Autodesk Inventor part; units mm, degrees
ref_plane "YZ Plane" through (0, 0, 0) normal (1, 0, 0) x (0, 1, 0)
ref_plane "XZ Plane" through (0, 0, 0) normal (0, 1, 0) x (-1, 0, 0)
ref_plane "XY Plane" through (0, 0, 0) normal (0, 0, 1) x (1, 0, 0)
sketch "Sketch1" plane through (0, 0, 0) normal (0, 1, 0) x (-1, 0, 0)
  line L0 (44.45, 203.2) -> (-44.45, 203.2)
  line L1 (-44.45, 203.2) -> (-44.45, -203.2)
  line L2 (-44.45, -203.2) -> (44.45, -203.2)
  line L3 (44.45, -203.2) -> (44.45, 203.2)
  line L4 (44.45, 203.2) -> (-44.45, -203.2) construction
  line L5 (-44.45, 203.2) -> (44.45, -203.2) construction
  line L6 (-44.45, 203.2) -> (-20.955, 203.2)
  line L7 (-20.955, 203.2) -> (-20.955, 88.9) construction
  line L8 (-44.45, 88.9) -> (-44.45, 203.2)
  circle A0 centre (-20.955, 88.9) radius 15.494 construction
  line L9 (44.45, 203.2) -> (44.45, 111.6492)
  line L10 (44.45, 203.2) -> (44.45, 38.1)
  line L11 (44.45, 38.1) -> (22.225, 38.1) construction
  circle A1 centre (22.225, 38.1) radius 12.065 construction
  line L12 (-66.675, 88.9) -> (0, 88.9) construction
  line L13 (0, 88.9) -> (0, 203.2) construction
  line L14 (0, 203.2) -> (-66.675, 203.2)
  line L15 (-66.675, 203.2) -> (-66.675, 88.9) construction
  line L16 (-66.675, 203.2) -> (-66.675, 209.55) construction
  line L17 (-66.675, 209.55) -> (32.5679, 44.312) construction
  circle A2 centre (-20.955, 104.394) radius 1.5
  circle A3 centre (-34.3732, 96.647) radius 1.5
  circle A4 centre (-34.3732, 81.153) radius 1.5
  circle A5 centre (-20.955, 73.406) radius 1.5
  circle A6 centre (-7.5368, 81.153) radius 1.5
  circle A7 centre (-7.5368, 96.647) radius 1.5
  circle A8 centre (-20.955, 88.9) radius 7.112 construction
  circle A9 centre (-28.067, 88.9) radius 5.9944
  line L18 (-20.955, 88.9) -> (-20.955, 152.4) construction
  circle A10 centre (-20.955, 152.4) radius 8.001 construction
  circle A11 centre (-20.955, 152.4) radius 4.0005
  circle A12 centre (-20.955, 160.401) radius 1.85
  line L19 (42.545, 152.4) -> (-20.955, 152.4) construction
  circle A13 centre (-28.956, 152.4) radius 1.85
  line L20 (-20.955, 215.9) -> (-20.955, 152.4) construction
  circle A14 centre (-20.955, 144.399) radius 1.85
  line L21 (-84.455, 152.4) -> (-20.955, 152.4) construction
  circle A15 centre (-12.954, 152.4) radius 1.85
  line L22 (44.45, 0) -> (-44.45, 0) construction
  circle A16 centre (22.225, 38.1) radius 2.9766
  circle A17 centre (22.225, -38.1) radius 2.9766
  circle A18 centre (-33.8743, 119.8397) radius 12.065 construction
  circle A19 centre (-33.8743, 119.8397) radius 2.9766
  circle A20 centre (-20.955, 152.4) radius 50.8 construction
  line L23 (32.5679, 44.312) -> (22.7595, 60.6429) construction
  line L24 (22.7595, 60.6429) -> (17.8553, 68.8083) construction
  line L25 (15.6729, 78.6085) -> (25.4813, 62.2776)
  line L26 (25.4813, 62.2776) -> (20.0377, 59.0081)
  line L27 (20.0377, 59.0081) -> (10.2292, 75.339)
  line L28 (10.2292, 75.339) -> (15.6729, 78.6085)
  line L29 (15.6729, 78.6085) -> (20.0377, 59.0081) construction
  line L30 (25.4813, 62.2776) -> (10.2292, 75.339) construction
  line L31 (-3.944, 111.2702) -> (5.8645, 94.9394)
  line L32 (-9.3876, 108.0008) -> (-3.944, 111.2702)
  line L33 (5.8645, 94.9394) -> (0.4208, 91.6699)
  line L34 (0.4208, 91.6699) -> (-9.3876, 108.0008)
  line L35 (-23.5608, 143.932) -> (-13.7524, 127.6011)
  line L36 (-29.0044, 140.6625) -> (-23.5608, 143.932)
  line L37 (-13.7524, 127.6011) -> (-19.196, 124.3316)
  line L38 (-19.196, 124.3316) -> (-29.0044, 140.6625)
  circle A21 centre (-20.955, -104.394) radius 1.5
  circle A22 centre (-34.3732, -81.153) radius 1.5
  circle A23 centre (-7.5368, -81.153) radius 1.5
  circle A24 centre (-28.067, -88.9) radius 5.9944
  circle A25 centre (-20.955, -152.4) radius 4.0005
  circle A26 centre (-28.956, -152.4) radius 1.85
  circle A27 centre (-12.954, -152.4) radius 1.85
  circle A28 centre (22.225, -38.1) radius 2.9766
  circle A29 centre (-33.8743, -119.8397) radius 2.9766
  circle A30 centre (-29.2932, -53.9743) radius 3.175
  circle A31 centre (-28.067, 88.9) radius 31.75 construction
  line L39 (-28.067, 88.9) -> (-44.45, 88.9) construction
  line L40 (-44.45, 88.9) -> (-44.45, 12.7)
  line L41 (44.45, 203.2) -> (34.925, 203.2)
  line L42 (34.925, 203.2) -> (34.925, 193.675) construction
  line L43 (34.925, 193.675) -> (44.45, 193.675) construction
  line L44 (44.45, 193.675) -> (44.45, 203.2)
  circle A32 centre (34.925, 193.675) radius 3.175
  line L45 (-44.45, 0) -> (-31.75, 0)
  circle A33 centre (-31.75, 0) radius 3.175
  circle A34 centre (34.925, -193.675) radius 3.175
  line L46 (-44.45, 0) -> (-19.455, 0) construction
  line L47 (-16.28, -76.0639) -> (-22.63, -76.0639) construction
  line L48 (-22.63, -76.0639) -> (-22.63, 51.9267) construction
  line L49 (-22.63, 51.9267) -> (-16.28, 51.9267) construction
  line L50 (-16.28, 51.9267) -> (-16.28, -76.0639) construction
  line L51 (-16.28, -63.9953) -> (-22.63, 63.9953) construction
  line L52 (-22.63, -63.9953) -> (-16.28, 63.9953) construction
  line L53 (-16.28, 51.9267) -> (-22.63, -76.0639) construction
  line L54 (-22.63, 51.9267) -> (-16.28, -76.0639) construction
  line L55 (-16.28, -2.5436) -> (-22.63, -2.5436)
  line L56 (-22.63, -2.5436) -> (-22.63, -21.5936)
  line L57 (-22.63, -21.5936) -> (-16.28, -21.5936)
  line L58 (-16.28, -21.5936) -> (-16.28, -2.5436)
  line L59 (-16.28, -2.5436) -> (-22.63, -21.5936) construction
  line L60 (-22.63, -2.5436) -> (-16.28, -21.5936) construction
  line L61 (-16.28, -40.6436) -> (-22.63, -40.6436)
  line L62 (-16.28, -59.6936) -> (-16.28, -40.6436)
  line L63 (-22.63, -40.6436) -> (-22.63, -59.6936)
  line L64 (-22.63, -59.6936) -> (-16.28, -59.6936)
  line L65 (-16.28, 35.5564) -> (-22.63, 35.5564)
  line L66 (-16.28, 16.5064) -> (-16.28, 35.5564)
  line L67 (-22.63, 35.5564) -> (-22.63, 16.5064)
  line L68 (-22.63, 16.5064) -> (-16.28, 16.5064)
  line L69 (-16.28, -2.5436) -> (-22.63, -2.5436)
  line L70 (-16.28, -21.5936) -> (-16.28, -2.5436)
  line L71 (-22.63, -2.5436) -> (-22.63, -21.5936)
  line L72 (-22.63, -21.5936) -> (-16.28, -21.5936)
  point P0 (0, 0)
  point P1 (-19.455, -12.0686)
  dimension "d4" = 30.988
  dimension "d7" = 24.13
  dimension "d16" = 14.224
  dimension "d19" = 16.002
  dimension "d0" = 88.9
  dimension "d1" = 406.4
  dimension "d2" = 114.3
  dimension "d3" = 23.495
  dimension "d5" = 165.1
  dimension "d6" = 22.225
  dimension "d10" = 6.35
  dimension "d14" = 360
  dimension "d17" = 11.9888
  dimension "d18" = 63.5
  dimension "d20" = 8.001
  dimension "d21" = 3.7
  dimension "d24" = 360
  dimension "d26" = 5.9531
  dimension "d27" = 24.13
  dimension "d28" = 5.9531
  dimension "d29" = 101.6
  dimension "d32" = 19.05
  dimension "d33" = 9.525
  dimension "d34" = 6.35
  dimension "d37" = 38.1
  dimension "d48" = 63.5
  dimension "d50" = 9.525
  dimension "d51" = 9.525
  dimension "d52" = 6.35
  dimension "d53" = 12.7
  dimension "d54" = 6.35
  dimension "d57" = 6.35
  dimension "d58" = 127.9906
  dimension "d59" = 6.35
  dimension "d60" = 19.05
  dimension "d63" = 38.1
  dimension "d66" = 38.1
extrude "Extrusion5" add sketch "Sketch1" along normal blind 6.35 contours L3 L2 L1 L0 | A2 | A4 | A6 | A12 | A14
properties part number "ChassisOutide10"
Read the model definition and answer for the solid it produces. Units are mm, in the model's axes. A direction names the side the tool comes from. Give positions to 0.01 mm unless a question says otherwise; leave off trailing zeros. Write each loop counter-clockwise with the first axis right and the second up, starting at its lowest first coordinate (ties: lowest second). Pieces come first, ordered by that corner, then holes. Notation, with made-up numbers: (48.25, 61.25) - (61.25, 61.25) arc R17 ccw to (61.25, 76.25) - close; hole circle Ø3 at (-37.75, 73). An arc over 180 degrees is marked (long way). Use CSV: the item, a comma, the result in double quotes. Start each with the question number.
Item 1: Consider line 1 (X direction, y = 3, z = 119.5); line 2 (X direction, y = 1.75, z = -50.5); line 3 (Z direction, x = 8, y = 3). Determine where each line is inside the solid, lowest interval first.
Item 2: The part is cut by section B-B, the plane y = 4. Count the separate pieces of the cut face and the enclosed holes in it, and give its area (3 significant figures).
Item 3: A flat-ended cylindrical pin translates along its axis: P1, Ø2.5, axis at x = 34.37, z = 96.65, coming from the -Y side. Find the tip coordinate at first contact, or state that the pin passes through.
Item 4: The part is cut by section A-A, the plane z = -88.9. Give the vertices of the cut face in (x, y).
Item 5: The mould has two halves that part along Z. Classify faces 1 (the flat face through (22.63, 3, -12)), 2 (the flat face through (22.63, 3, -50)), 3 (the flat face through (1, 3, -203.2)), 4 (the flat face through (1, 6.35, 3)): pulls with the +Z half, pulls with the -Z half, needs draft (parallel to the pull), parting line crosses it, or undercut.
Item 6: For faces 5 (the flat face through (19, 3, -59.694)), 6 (the flat face through (-44.45, 3, -3)), determine the directions among +Z, -Z, +X, -X, +Y, -Y from which every point of the face is accessible in a straight line to the end or side of a thin tool.
Taken from the geometry:
1,line 1,"-44.45 to 30.92, 36.83 to 44.45"
1,line 2,"-44.45 to 16.28, 22.63 to 44.45"
1,line 3,"-203.2 to -82.58, -79.73 to 95.22, 98.07 to 105.69, 108.83 to 203.2"
2,separate pieces,"1"
2,enclosed holes,"28"
2,area,"34,800 mm2"
3,P1,"through"
4,outline,"(-44.45, 0) - (22.07, 0) - (22.07, 6.35) - (-44.45, 6.35) - close; (34.06, 0) - (44.45, 0) - (44.45, 6.35) - (34.06, 6.35) - close"
5,face 1,"undercut"
5,face 2,"undercut"
5,face 3,"pulls with the -Z half"
5,face 4,"needs draft"
6,face 5,"+Y, -Y"
6,face 6,"+Z, -Z, -X, +Y, -Y"
